For this review, use the dimensioned drawing (mm, ordinates from the lowest corner) and the shaded views. A direction names the side the tool comes from. Coordinates: 2 decimals unless noted, no trailing zeros. Order: outer loops, then holes, each group sorted by start corner. A loop starts at its lowest first (then second) coordinate and runs counter-clockwise, first axis right, second up. Notation, with made-up numbers: M -22,33 L 15,33 A20 cw 15,45 Z; hole C -36.75,69 d9. An arc over 180 degrees is marked long. Write each question's results on one line, items separated by ' | '.
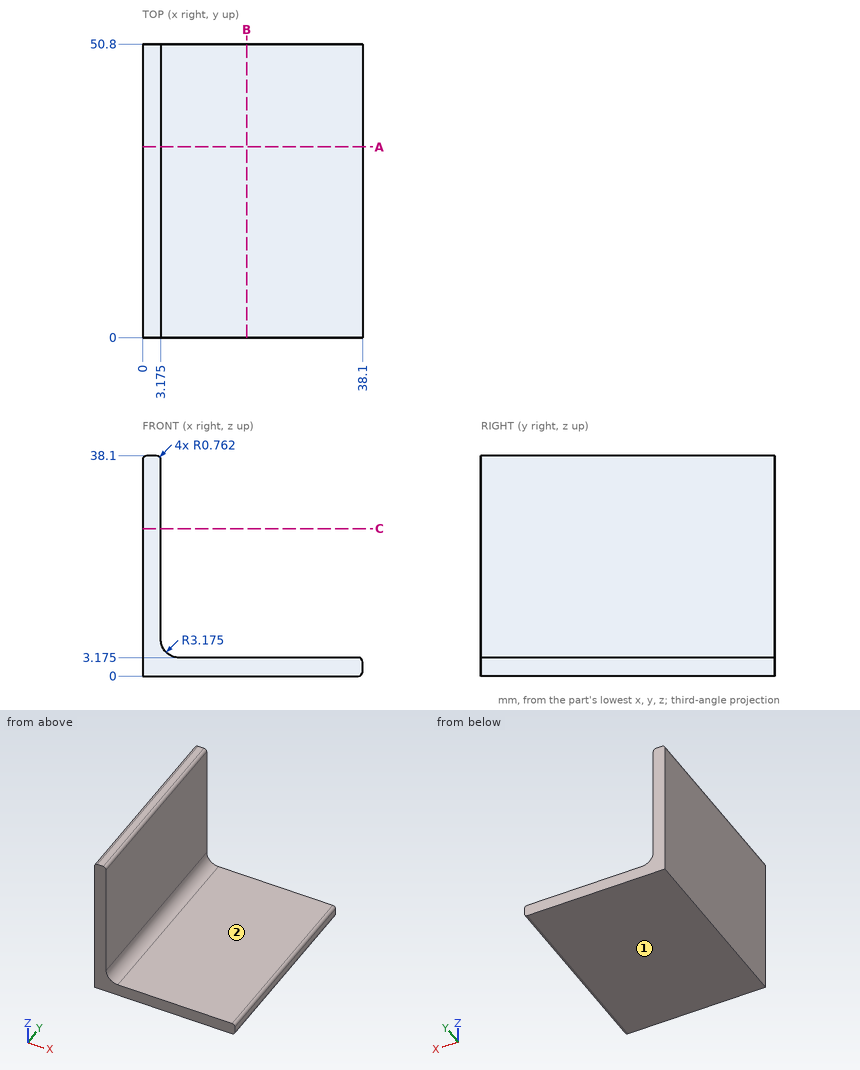
1) For the marked faces 1 and 2, list the 3-axis set-ups (+Z, -Z, +X, -X, +Y, -Y) from which the entire face can be reached by the end or side of a thin tool; tool diameter is ignored.
Solutions:
face 1: -Z, +X, -X, +Y, -Y | face 2: +Z, +X, +Y, -Y
2) Take a section at A-A on y = 33. State the section outline as (x, z) points (3 decimals).
Solutions:
outline: M 0,0 L 37.338,0 A0.762 ccw 38.1,0.762 L 38.1,2.413 A0.762 ccw 37.338,3.175 L 6.35,3.175 A3.175 cw 3.175,6.35 L 3.175,37.338 A0.762 ccw 2.413,38.1 L 0.762,38.1 A0.762 ccw 0,37.338 Z
3) For pin 1 (4 mm diameter, centred on y = 43.5, z = 16.5, fed in from +X) (3 decimals); pin 2 (8 mm diameter, centred on x = 9, z = 23.5, fed in from +Y); pin 3 (10 mm diameter, centred on x = 27, y = 14, fed in from +Z) (3 decimals), all flat-tipped, find the tip position at first contact; note any pin that passes through.
Solutions:
pin 1: x = 3.175 | pin 2: through | pin 3: z = 3.175
4) Take a section at B-B on x = 18. State the section outline as (y, z) points (3 decimals).
Solutions:
outline: M 0,0 L 50.8,0 L 50.8,3.175 L 0,3.175 Z
5) To check wall thickness, follow line 1 along X through (y, z) = (29, 9.5) (3 decimals). State the ranges of the line that lie inside material, in increasing order.
Solutions:
line 1: 0 to 3.175
6) Take a section at C-C on z = 25.5. State the section outline as (x, y) points (3 decimals), plus the area to 3 significant figures.
Solutions:
outline: M 0,0 L 3.175,0 L 3.175,50.8 L 0,50.8 Z | area: 161 mm2
